from build123d import *

# Parameters (mm, degrees)
F1_DEPTH = 25


with BuildPart() as f1:
    # F0 (on Front) → F1 (new body)
    with BuildSketch(Plane.XZ):
        with BuildLine():
            ThreePointArc((-123.001458, 122.857143), (-137.142857, 123.001458), (-136.998542, 137.142857))
            ThreePointArc((-136.998542, 137.142857), (-136.890306, 147.748907), (-147.496355, 147.857143))
            ThreePointArc((-147.496355, 147.857143), (-154.846467, 132.766417), (-150.995626, 116.428571))
            ThreePointArc((-150.995626, 116.428571), (-148.270306, 112.935536), (-144.97119, 109.978425))
            Line((-144.97119, 109.978425), (-19.94447, 16.489339))
            Line((-19.94447, 16.489339), (0, 15))
            Line((0, 15), (0, 245))
            Line((0, 245), (-19.94447, 243.510661))
            Line((-19.94447, 243.510661), (-110.097784, 176.098264))
            ThreePointArc((-110.097784, 176.098264), (-117.370449, 165.507995), (-116.70046, 152.678476))
            ThreePointArc((-116.70046, 152.678476), (-115.341488, 136.814996), (-123.001458, 122.857143))
        make_face()
    extrude(amount=F1_DEPTH)


solid = f1.part
Geometry check sheet. Reference: the model listing, model coordinates, mm. A direction names the side the tool comes from. Round coordinates to 2 decimals unless told otherwise and drop trailing zeros. Loops run counter-clockwise (first coordinate to the right, second up) from the corner with the lowest first, then second, coordinate; pieces in that order, holes last. Notation, with made-up numbers: (37.5, -8) -> (89.5, -8) arc R34 cw to (89.5, 31) -> close; hole circle Ø6 at (80.25, -6). An arc over 180 degrees is marked (long way). Answer as a JSON object with one key per item and string values. Group by question number.
Item 1: Cross-section at D-D, the plane z = 207. Record the cut outline in (x, y), plus the area to 3 significant figures.
Item 2: Thickness scan on line 1 along X through (y, z) = (-19, 24.5); line 2 along Z through (x, y) = (-23, -7); line 3 along Z through (x, y) = (-38.5, -19.5). Record the ranges inside material, lowest first.
Item 3: Cross-section at C-C, the plane x = -107. Record the cut outline in (y, z).
Item 4: Cross-section at A-A, the plane z = 130. Record the cut outline in (x, y), plus the area to 3 significant figures.
Item 5: Depth check by flat-ended pin: pin 1 Ø3 at (y, z) = (-10.5, 81) entering from -X; pin 2 Ø5 at (y, z) = (-9, 108.5) entering from -X; pin 3 Ø2 at (y, z) = (-10, 67) entering from -X. Enter the tip coordinate at first touch or a pass-through.
Item 6: Cross-section at B-B, the plane y = -18. Record the cut outline in (x, z), plus the area to 3 significant figures.
Item 7: Set-up check for faces 1 (the face through (-115.296, -12.325, 137.036)), 2 (the face through (-10.112, -12.325, 15.755)): record each of +Z, -Z, +X, -X, +Y, -Y from which the full face is reachable in a straight line by a thin tool's end or side.
Determined:
{
 "1": {"outline": "(-68.77, -25) -> (0, -25) -> (0, 0) -> (-68.77, 0) -> close", "area": "1,720 mm²"},
 "2": {"line 1": "x = -30.66 to 0", "line 2": "z = 18.77 to 241.23", "line 3": "z = 30.36 to 229.64"},
 "3": {"outline": "(-25, 81.59) -> (0, 81.59) -> (0, 178.41) -> (-25, 178.41) -> close"},
 "4": {"outline": "(-155, -25) -> (-140, -25) -> (-140, 0) -> (-155, 0) -> close; (-117.75, -25) -> (0, -25) -> (0, 0) -> (-117.75, 0) -> close", "area": "3,320 mm²"},
 "5": {"pin 1": "stops at x = -108.22", "pin 2": "stops at x = -146.25", "pin 3": "stops at x = -88.83"},
 "6": {"outline": "(-151, 116.43) arc R25 ccw to (-144.97, 109.98) -> (-19.94, 16.49) -> (0, 15) -> (0, 245) -> (-19.94, 243.51) -> (-110.1, 176.1) arc R20 ccw to (-116.7, 152.68) arc R27.5 cw to (-123, 122.86) arc R10 cw to (-137, 137.14) arc R7.5 ccw to (-147.5, 147.86) arc R25 ccw to start", "area": "20,600 mm²"},
 "7": {"face 1": "+Y, -Y", "face 2": "-Z, -X, +Y, -Y"}
}
